```python
from build123d import *

# Parameters (mm, degrees)
F1_ANGLE  = 180
F2_W      = 10.16
F2_H      = 10.16
F3_DEPTH  = 7.62
F4_R      = 3.2385
F5_DEPTH  = 25.4
F6_W      = 10.16
F6_H      = 10.16
F7_DEPTH  = 7.62
F8_R      = 3.2385
F9_DEPTH  = 25.4
F11_DEPTH = 25.4
F12_DEPTH = 25.4
F13_DEPTH = 25.4
F14_R     = 5.08


with BuildPart() as f1:
    # F0 (on Front) → F1 (revolve)
    with BuildSketch(Plane.XZ):
        with BuildLine():
            Line((-62.4678657544, 68.8326101213), (-66.2778657544, 68.8326101213))
            Line((-66.2778657544, 68.8326101213), (-66.2778657544, -7.3673898787))
            Line((-66.2778657544, -7.3673898787), (-56.3942688751, -7.3673898787))
            Line((-56.3942688751, -7.3673898787), (-5.3178657544, -7.3673898787))
            Line((-5.3178657544, -7.3673898787), (-5.3178657544, -2.4929920513))
            ThreePointArc((-5.3178657544, -2.4929920513), (-7.1777376938, 1.9971360092), (-11.6678657544, 3.8570079487))
            Line((-11.6678657544, 3.8570079487), (-49.7678657544, 3.8570079487))
            ThreePointArc((-49.7678657544, 3.8570079487), (-54.2579938149, 5.7168798881), (-56.1178657544, 10.2070079487))
            Line((-56.1178657544, 10.2070079487), (-56.1178657544, 62.4826101213))
            ThreePointArc((-56.1178657544, 62.4826101213), (-57.9777376938, 66.9727381818), (-62.4678657544, 68.8326101213))
        make_face()
    revolve(axis=Axis((-122.1578657544, 0, 30.7326101213), (0, 0, -1)), revolution_arc=F1_ANGLE)

    # F2 (on face) → F3 (join)
    with BuildSketch(Plane(origin=(0, 0, 0), x_dir=(-1, 0, 0), z_dir=(0, 1, 0))):
        with Locations((61.1978657544, 31.264809035)):
            Rectangle(F2_W, F2_H)
        with Locations((51.0378657544, 31.264809035)):
            Rectangle(F2_W, F2_H)
    extrude(amount=-F3_DEPTH)

    # F4 (on face) → F5 (cut)
    with BuildSketch(Plane(origin=(0, 0, 0), x_dir=(-1, 0, 0), z_dir=(0, 1, 0))):
        with Locations((51.0378657544, 31.264809035)):
            Circle(F4_R)
    extrude(amount=-F5_DEPTH, mode=Mode.SUBTRACT)

    # F6 (on face) → F7 (join)
    with BuildSketch(Plane(origin=(0, 0, 0), x_dir=(-1, 0, 0), z_dir=(0, 1, 0))):
        with Locations((183.1178657544, 31.264809035)):
            Rectangle(F6_W, F6_H)
        with Locations((193.2778657544, 31.264809035)):
            Rectangle(F6_W, F6_H)
    extrude(amount=-F7_DEPTH)

    # F8 (on face) → F9 (cut)
    with BuildSketch(Plane(origin=(0, 0, 0), x_dir=(-1, 0, 0), z_dir=(0, 1, 0))):
        with Locations((193.2778657544, 31.264809035)):
            Circle(F8_R)
    extrude(amount=-F9_DEPTH, mode=Mode.SUBTRACT)

    # F10 (on face) → F11 (cut)
    with BuildSketch(Plane.XY.offset(3.8570079487)):
        with BuildLine():
            ThreePointArc((-201.347260479, -45.8019683397), (-202.1444682095, -44.3924875908), (-202.9165913892, -42.9691106405))
            ThreePointArc((-202.9165913892, -42.9691106405), (-204.1518837491, -47.4212183397), (-199.6785992012, -48.5774776245))
            ThreePointArc((-199.6785992012, -48.5774776245), (-200.5252182095, -47.1971108609), (-201.347260479, -45.8019683397))
        make_face()
        with BuildLine():
            ThreePointArc((-198.5426372088, -44.1827183397), (-200.4814096168, -42.6813619028), (-202.9165913892, -42.9691106405))
            ThreePointArc((-202.9165913892, -42.9691106405), (-202.1444682095, -44.3924875908), (-201.347260479, -45.8019683397))
            Line((-201.347260479, -45.8019683397), (-198.5426372088, -44.1827183397))
        make_face()
        with BuildLine():
            Line((-198.5426372088, -44.1827183397), (-201.347260479, -45.8019683397))
            ThreePointArc((-201.347260479, -45.8019683397), (-200.5252182095, -47.1971108609), (-199.6785992012, -48.5774776245))
            ThreePointArc((-199.6785992012, -48.5774776245), (-198.5284094898, -47.3963212966), (-198.108760479, -45.8019683397))
            ThreePointArc((-198.108760479, -45.8019683397), (-198.2191096905, -44.9637828622), (-198.5426372088, -44.1827183397))
        make_face()
        with BuildLine():
            ThreePointArc((-122.1578657544, -91.521986701), (-123.7771157544, -91.5076484732), (-125.3958579423, -91.4646382865))
            ThreePointArc((-125.3958579423, -91.4646382865), (-122.1865410857, -94.7603597455), (-118.9193657544, -91.521986701))
            ThreePointArc((-118.9193657544, -91.521986701), (-118.9194927099, -91.4933113696), (-118.9198735664, -91.4646382865))
            ThreePointArc((-118.9198735664, -91.4646382865), (-120.5386157544, -91.5076484732), (-122.1578657544, -91.521986701))
        make_face()
        with BuildLine():
            ThreePointArc((-122.1578657544, -88.283486701), (-124.4274647729, -89.2118346399), (-125.3958579423, -91.4646382865))
            ThreePointArc((-125.3958579423, -91.4646382865), (-123.7771157544, -91.5076484732), (-122.1578657544, -91.521986701))
            Line((-122.1578657544, -91.521986701), (-122.1578657544, -88.283486701))
        make_face()
        with BuildLine():
            ThreePointArc((-118.9198735664, -91.4646382865), (-119.8882667358, -89.2118346399), (-122.1578657544, -88.283486701))
            Line((-122.1578657544, -88.283486701), (-122.1578657544, -91.521986701))
            ThreePointArc((-122.1578657544, -91.521986701), (-120.5386157544, -91.5076484732), (-118.9198735664, -91.4646382865))
        make_face()
        with BuildLine():
            ThreePointArc((-39.7299710298, -45.8019683397), (-40.178295372, -44.1579482521), (-41.3991401196, -42.9691106405))
            ThreePointArc((-41.3991401196, -42.9691106405), (-42.1712632993, -44.3924875908), (-42.9684710298, -45.8019683397))
            ThreePointArc((-42.9684710298, -45.8019683397), (-43.7905132993, -47.1971108609), (-44.6371323075, -48.5774776245))
            ThreePointArc((-44.6371323075, -48.5774776245), (-41.3741180729, -48.6208193289), (-39.7299710298, -45.8019683397))
        make_face()
        with BuildLine():
            Line((-42.9684710298, -45.8019683397), (-45.7730942999, -44.1827183397))
            ThreePointArc((-45.7730942999, -44.1827183397), (-46.1039209105, -46.6124227157), (-44.6371323075, -48.5774776245))
            ThreePointArc((-44.6371323075, -48.5774776245), (-43.7905132993, -47.1971108609), (-42.9684710298, -45.8019683397))
        make_face()
        with BuildLine():
            ThreePointArc((-42.9684710298, -45.8019683397), (-42.1712632993, -44.3924875908), (-41.3991401196, -42.9691106405))
            ThreePointArc((-41.3991401196, -42.9691106405), (-43.834321892, -42.6813619028), (-45.7730942999, -44.1827183397))
            Line((-45.7730942999, -44.1827183397), (-42.9684710298, -45.8019683397))
        make_face()
    extrude(amount=-F11_DEPTH, mode=Mode.SUBTRACT)

    # F12 (add): a face of the model
    f12_faces = [f1.faces().sort_by_distance(p)[0] for p in [
        (-193.2036113422, -3.8371570424, 26.184809035),
    ]]
    extrude(f12_faces, amount=F12_DEPTH)

    # F13 (add): a face of the model
    f13_faces = [f1.faces().sort_by_distance(p)[0] for p in [
        (-51.1121201665, -3.8371570424, 26.184809035),
    ]]
    extrude(f13_faces, amount=F13_DEPTH)

    # F14
    f14_edges = [f1.edges().sort_by_distance(p)[0] for p in [
        (-198.357866, -3.81, 3.857008),
        (-188.087501, -3.816378, 36.344809),
        (-45.957866, -3.81, 3.857008),
        (-56.22823, -3.816378, 36.344809),
    ]]
    fillet(f14_edges, radius=F14_R)


solid = f1.part
```
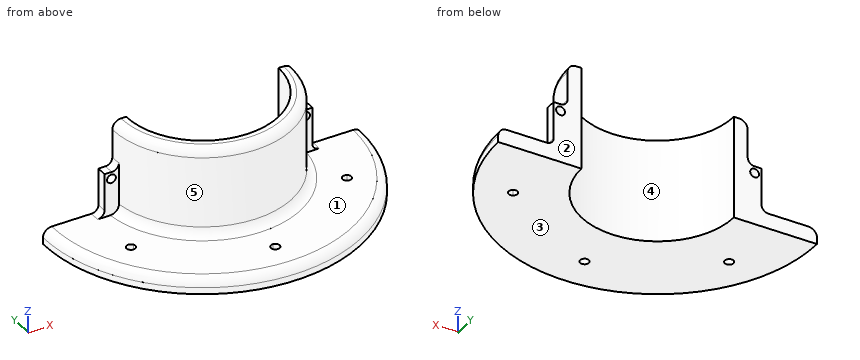
For this review, take the finished solid that the model builds, in its own axes (mm). Face numbers are marked on the shaded views. A direction names the side the tool comes from. Round coordinates to 2 decimals unless told otherwise and drop trailing zeros. Write each loop counter-clockwise with the first axis right and the second up, starting at its lowest first coordinate (ties: lowest second). Pieces come first, ordered by that corner, then holes. Notation, with made-up numbers: (-18, 60) - (9, 60) arc R20 ccw to (9, 93) - close; hole circle Ø7 at (-13.5, 28). An arc over 180 degrees is marked (long way). Put each result on its own line as item: value.
Q1. Machinability: for the marked faces 4 and 5, which of the approach directions +Z, -Z, +X, -X, +Y, -Y give a long, thin tool a straight path to every point of the face, cutting with its end or side? Answer none if there is none.
Solved:
face 4: +Z, -Z, +Y
face 5: +Z, -Y
Q2. Mouldability with a two-part tool opening along Z and no side actions: class the marked faces 1, 2 and 3 as released by +Z, released by -Z, zero draft, split by the parting line, or undercut.
Solved:
face 1: released by +Z
face 2: zero draft
face 3: released by -Z
Q3. Wall thickness on probe 1 along Z at (x, y) = (-152.5, -102); probe 2 along Y at (x, z) = (-124, 25); probe 3 along X at (y, z) = (-35, 22.5): over which ranges is each line inside the solid? List them lowest first.
Solved:
probe 1: z = -7.37 to 3.86
probe 2: y = -66.01 to -55.85
probe 3: x = -178.16 to -165.72, -78.6 to -66.16
Q4. We need section B-B (z = 51.5). Give the boundary of the cut face in (x, y), and give its area (3 significant figures).
Solved:
outline: (-188.2, 0) arc R66.04 ccw to (-56.12, 0) - (-66.28, 0) arc R55.88 cw to (-178.04, 0) - close
area: 1,950 mm2
Q5. We need section A-A (z = 1.5). Give the boundary of the cut face in (x, y).
Solved:
outline: (-237.59, 0) arc R115.43 ccw to (-6.73, 0) - (-66.28, 0) arc R55.88 cw to (-178.04, 0) - close; hole circle Ø6.48 at (-201.35, -45.8); hole circle Ø6.48 at (-122.16, -91.52); hole circle Ø6.48 at (-42.97, -45.8)
Q6. Insertion check: pin 1 Ø3 at (x, y) = (-44, -21) entering from +Z; pin 2 Ø5 at (x, z) = (-132.5, 41.5) entering from -Y; pin 3 Ø7.5 at (x, z) = (-51.04, 31.26) entering from -Y. Each pin has a flat end and moves straight along its axis. Give the tip position at first contact, or say it passes through.
Solved:
pin 1: stops at z = 3.86
pin 2: stops at y = -65.57
pin 3: stops at y = -7.62
